```python
from build123d import *

# Parameters (mm, degrees)
F0_W     = 59
F0_H     = 8
F0_H_2   = 98
F0_R     = 2.15
F1_DEPTH = 82
F2_W     = 62.2
F2_H     = 98
F3_DEPTH = 25
F4_DEPTH = 125.3
F5_R     = 2.1
F5_R_2   = 2.65
F5_W     = 62.2
F5_H     = 10
F6_DEPTH = 20.8
F7_R     = 7.9669047558
F8_R     = 11.1053823869
F9_R     = 5


with BuildPart() as f1:
    # F0 (on Right) → F1 (new body)
    with BuildSketch(Plane.YZ):
        with Locations((21.5, 62.4624560177)):
            Rectangle(F0_W, F0_H)
        with Locations((21.5, 9.4624560177)):
            Rectangle(F0_W, F0_H_2)
        with BuildLine():
            ThreePointArc((0, -33.7875439823), (-2.25, -31.5375439823), (0, -29.2875439823))
            Line((0, -29.2875439823), (0, 9.3124560177))
            ThreePointArc((0, 9.3124560177), (-1.5202795796, 12.9827355973), (2.15, 11.4624560177))
            ThreePointArc((2.15, 11.4624560177), (2.117336669, 11.0891124357), (2.0203391347, 10.7271127096))
            Line((2.0203391347, 10.7271127096), (38.292474297, -2.4748648228))
            ThreePointArc((38.292474297, -2.4748648228), (40.7974910935, -1.028592701), (42.6567826938, -3.2444101453))
            ThreePointArc((42.6567826938, -3.2444101453), (42.6226001381, -3.635118545), (42.5210910906, -4.0139554678))
            ThreePointArc((42.5210910906, -4.0139554678), (25.9543337449, -25.6041739863), (0, -33.7875439823))
        make_face(mode=Mode.SUBTRACT)
        with Locations((43, -31.5375439823)):
            Circle(F0_R, mode=Mode.SUBTRACT)
        with BuildLine():
            Line((0, 9.3124560177), (0, -29.2875439823))
            ThreePointArc((0, -29.2875439823), (23.3732397813, -21.917989787), (38.292474297, -2.4748648228))
            Line((38.292474297, -2.4748648228), (2.0203391347, 10.7271127096))
            ThreePointArc((2.0203391347, 10.7271127096), (1.2331893382, 9.7012791225), (0, 9.3124560177))
        make_face()
    extrude(amount=F1_DEPTH)

    # F2 (on face) → F3 (join)
    with BuildSketch(Plane.XZ.offset(8)):
        with Locations((41, 9.4624560177)):
            Rectangle(F2_W, F2_H)
    extrude(amount=F3_DEPTH)

    # F4 (cut): a face of the model
    f4_faces = [f1.faces().sort_by_distance(p)[0] for p in [
        (41, -33, 9.4624560177),
    ]]
    extrude(f4_faces, amount=-F4_DEPTH, mode=Mode.SUBTRACT)

    # F5 (on face) → F6 (cut)
    with BuildSketch(Plane(origin=(0, 0, 58.4624560177), x_dir=(1, 0, 0), z_dir=(0, 0, -1))):
        with Locations((41, -22)):
            Circle(F5_R)
        with Locations((53.5, -22)):
            Circle(F5_R_2)
        with Locations((34.5, -27)):
            Circle(F5_R_2)
        with Locations((36, -15.5)):
            Circle(F5_R_2)
        with Locations((41, -34.5)):
            Circle(F5_R_2)
        with Locations((41, -46)):
            Rectangle(F5_W, F5_H)
    extrude(amount=-F6_DEPTH, mode=Mode.SUBTRACT)

    # F7
    f7_edges = [f1.edges().sort_by_distance(p)[0] for p in [
        (9.9, 16.5, 58.462456),
        (72.1, 16.5, 58.462456),
    ]]
    fillet(f7_edges, radius=F7_R)

    # F8
    f8_edges = [f1.edges().sort_by_distance(p)[0] for p in [
        (4.95, -8, -39.537544),
        (4.95, 51, -39.537544),
        (77.05, 51, -39.537544),
        (77.05, -8, -39.537544),
    ]]
    fillet(f8_edges, radius=F8_R)

    # F9
    f9_edges = [f1.edges().sort_by_distance(p)[0] for p in [
        (9.9, 41, 62.462456),
        (72.1, 41, 62.462456),
    ]]
    fillet(f9_edges, radius=F9_R)


solid = f1.part
```
Geometry check sheet. Reference: the model listing, model coordinates, mm. A direction names the side the tool comes from. Coordinates: 2 decimals unless noted, no trailing zeros. Loops run counter-clockwise (first coordinate to the right, second up) from the corner with the lowest first, then second, coordinate; pieces in that order, holes last. Notation, with made-up numbers: (42.5, 54) -> (99.5, 54) arc R20 ccw to (99.5, 87) -> close; hole circle Ø4 at (40.5, 54). An arc over 180 degrees is marked (long way). Put each result on its own line as item: value.
1) Tool access check on faces 1 (the cylindrical face through (4.88, -2.25, -31.59)), 2 (the cylindrical face through (69.828, 19.378, 56.067)), 3 (the cylindrical face through (11.33, 42.5, 60.14)). Record the directions out of +Z, -Z, +X, -X, +Y, -Y that give a thin tool (end or side, any length) a straight path to the whole face; none if there is none.
Result set:
face 1: +X, -X
face 2: -Z, +Y, -Y
face 3: +Z, -Z, +Y
2) Cross-section at C-C on y = 27. Record the boundary of the cut face in (x, z), plus the area to 3 significant figures.
Result set:
outline: (0, -39.54) -> (9.9, -39.54) -> (9.9, -24.85) -> (0, -24.85) -> close; (0, -19.06) -> (9.9, -19.06) -> (9.9, 50.5) arc R7.97 cw to (17.87, 58.46) -> (31.85, 58.46) -> (31.85, 66.46) -> (0, 66.46) -> close; (37.15, 58.46) -> (64.13, 58.46) arc R7.97 cw to (72.1, 50.5) -> (72.1, -19.06) -> (82, -19.06) -> (82, 66.46) -> (37.15, 66.46) -> close; (72.1, -39.54) -> (82, -39.54) -> (82, -24.85) -> (72.1, -24.85) -> close
area: 2,470 mm^2
3) Gauge pin test, flat ends, axial feed: pin 1 Ø2.5 at (y, z) = (0, 11.46) entering from -X; pin 2 Ø7 at (x, y) = (41, 34.5) entering from -Z; pin 3 Ø2.5 at (x, z) = (48, 61) entering from +Y. Record the tip position at first contact, or that the pin passes through.
Result set:
pin 1: passes through
pin 2: stops at z = 58.46
pin 3: stops at y = 41
4) Release check for a two-part mould opening along Z. For faces 4 (the cylindrical face through (12.296, 19.378, 56.191)), 5 (the cylindrical face through (76.981, 43.992, -33.445)), 6 (the flat face through (82, 21, 14)) record: released by +Z, released by -Z, zero draft, split by the parting line, or undercut.
Result set:
face 4: released by -Z
face 5: undercut
face 6: zero draft
5) Cross-section at A-A on x = 53.5. Record the boundary of the cut face in (y, z).
Result set:
outline: (-8, 58.46) -> (19.35, 58.46) -> (19.35, 66.46) -> (-8, 66.46) -> close; (24.65, 58.46) -> (41, 58.46) -> (41, 66.46) -> (24.65, 66.46) -> close
6) Cross-section at D-D on z = -22.5. Record the boundary of the cut face in (x, y), plus the area to 3 significant figures.
Result set:
outline: (0, -8) -> (9.9, -8) -> (9.9, 22.52) -> (0, 22.52) -> close; (0, 29.9) -> (9.9, 29.9) -> (9.9, 51) -> (0, 51) -> close; (72.1, -8) -> (82, -8) -> (82, 22.52) -> (72.1, 22.52) -> close; (72.1, 29.9) -> (82, 29.9) -> (82, 51) -> (72.1, 51) -> close
area: 1,020 mm^2
7) Thickness scan on line 1 (Y direction, x = 41, z = 61); line 2 (X direction, y = 1, z = 43); line 3 (X direction, y = 34.5, z = 61.5). Record the ranges inside material, lowest first.
Result set:
line 1: y = -8 to 19.9, 24.1 to 31.85, 37.15 to 41
line 2: x = 0 to 9.9, 72.1 to 82
line 3: x = 0 to 38.35, 43.65 to 82
8) Cross-section at B-B on z = 23. Record the boundary of the cut face in (x, y).
Result set:
outline: (0, -8) -> (9.9, -8) -> (9.9, 51) -> (0, 51) -> close; (72.1, -8) -> (82, -8) -> (82, 51) -> (72.1, 51) -> close
